Input: part model. Units: mm. Frame: model coordinates. Face numbers are marked on the shaded views. Round coordinates to 2 decimals unless told otherwise and drop trailing zeros. Loops run counter-clockwise (first coordinate to the right, second up) from the corner with the lowest first, then second, coordinate; pieces in that order, holes last. Notation, with made-up numbers: M 53,-34.75 L 74,-34.75 A18 cw 74,-5.75 Z; hole C 2,76 d2. An arc over 180 degrees is marked long. Return JSON: item names as keys, results as strings. Group by question number.
1) Mould query, pull axis X, two halves, no side actions, for the marked faces 1 and 2. Classes: +X half, -X half, draft (parallel to the pull), parting line (faces both ways), or undercut.
2) Contact query for flat-ended pins moving along their axis: P1, Ø20, axis at x = -6, y = 5, coming from the -Z side; P2, Ø1, axis at x = 5, y = -8.5, coming from the -Z side. Output: stop coordinate, or through.
3) Material intervals for line 1 (X direction, y = 0, z = 0.4); line 2 (Z direction, x = 2, y = -5), sorted ascending. Write a range as from..to.
4) Section D-D (y = -19.5). Output: boundary loops of the cut face in (x, z), plus the area to 3 significant figures.
5) Section A-A (z = 2.5). Output: boundary loops of the cut face in (x, y), plus the area to 3 significant figures.
6) Section B-B (y = 0). Output: boundary loops of the cut face in (x, z).
7) Section C-C (x = -20). Output: boundary loops of the cut face in (y, z).
Autodesk Fusion 360 part; units mm, degrees
sketch "Sketch1" plane through (0, 0, 0) normal (0, 0, 1) x (1, 0, 0)
  circle A0 centre (0, 0) radius 12.5
  line L0 (0, 0) -> (-25, 0)
  line L1 (-25, 25) -> (25, 25)
  line L2 (25, 25) -> (25, -25)
  line L3 (25, -25) -> (-25, -25)
  line L4 (-25, -25) -> (-25, 25)
  dimension "d1" = 25
extrude "Extrude1" add sketch "Sketch1" along normal blind 3 contours A0 | L1 L2 L3 L4
extrude "Extrude2" cut sketch "Sketch1" along normal blind 0.5 contours A0
fillet "Fillet1" radius 10 4 edges at (25, -25, 1.5) (25, 25, 1.5) (-25, 25, 1.5) (-25, -25, 1.5)
sketch "Sketch2" plane through (0, 0, 0) normal (0, 0, 1) x (1, 0, 0)
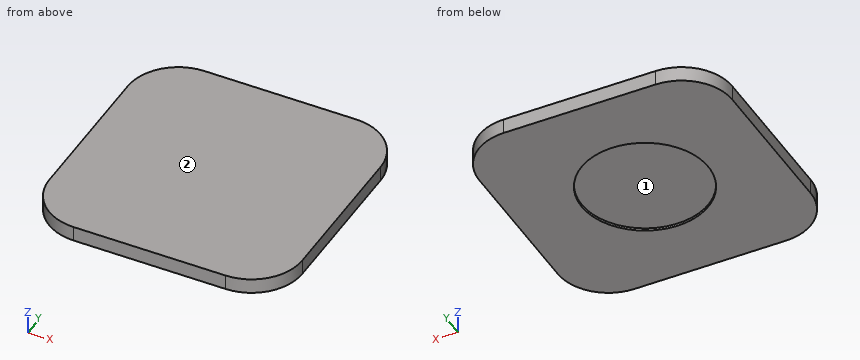
Returned:
{
 "1": {"face 1": "undercut", "face 2": "draft"},
 "2": {"P1": "stops at z = 0", "P2": "stops at z = 0.5"},
 "3": {"line 1": "x = -25..-12.5, 12.5..25", "line 2": "z = 0.5..3"},
 "4": {"outline": "M -23.93,0 L 23.93,0 L 23.93,3 L -23.93,3 Z", "area": "144 mm^2"},
 "5": {"outline": "M -25,-15 A10 ccw -15,-25 L 15,-25 A10 ccw 25,-15 L 25,15 A10 ccw 15,25 L -15,25 A10 ccw -25,15 Z", "area": "2,410 mm^2"},
 "6": {"outline": "M -25,0 L -12.5,0 L -12.5,0.5 L 12.5,0.5 L 12.5,0 L 25,0 L 25,3 L -25,3 Z"},
 "7": {"outline": "M -23.66,0 L 23.66,0 L 23.66,3 L -23.66,3 Z"}
}
